from build123d import *

# Parameters (mm, degrees)
SKETCH1_W           = 50.8
SKETCH1_H           = 76.2
SKETCH1_W_2         = 44.45
SKETCH1_H_2         = 69.85
BOSS_EXTRUDE1_DEPTH = 965.2
CUT_EXTRUDE1_REACH  = 969.287
SKETCH4_R           = 14.224
SKETCH5_R           = 2.50063
CUT_EXTRUDE2_DEPTH  = 3.175


with BuildPart() as part:
    # Sketch1 → Boss-Extrude1 (new body)
    with BuildSketch(Plane.XY):
        Rectangle(SKETCH1_W, SKETCH1_H)
        Rectangle(SKETCH1_W_2, SKETCH1_H_2, mode=Mode.SUBTRACT)
    extrude(amount=BOSS_EXTRUDE1_DEPTH)

    # Cut-Extrude1: up to this face of the body (flat: up to its plane)
    cut_extrude1_end = Plane(part.part.faces().sort_by_distance((-25.4, 0, 482.6))[0])
    # Sketch4 → Cut-Extrude1 (cut, up to the picked face)
    with BuildSketch(Plane(origin=(25.4, 0, 0), x_dir=(0, 0, -1), z_dir=(1, 0, 0)), mode=Mode.PRIVATE) as cut_extrude1_sk1:
        with Locations(Location((-703.246600733, 0, 0), (0, 0, 90))):
            Circle(SKETCH4_R)
    cut_extrude1_tool1 = split(extrude(cut_extrude1_sk1.sketch, amount=-CUT_EXTRUDE1_REACH, mode=Mode.PRIVATE), bisect_by=cut_extrude1_end, keep=Keep.BOTH, mode=Mode.PRIVATE)
    # Sketch4 → Cut-Extrude1 (cut, up to the picked face)
    with BuildSketch(Plane(origin=(25.4, 0, 0), x_dir=(0, 0, -1), z_dir=(1, 0, 0)), mode=Mode.PRIVATE) as cut_extrude1_sk2:
        with Locations(Location((-190.549048411, 0, 0), (0, 0, 90))):
            Circle(SKETCH4_R)
    cut_extrude1_tool2 = split(extrude(cut_extrude1_sk2.sketch, amount=-CUT_EXTRUDE1_REACH, mode=Mode.PRIVATE), bisect_by=cut_extrude1_end, keep=Keep.BOTH, mode=Mode.PRIVATE)
    # Sketch4 → Cut-Extrude1 (cut, up to the picked face)
    with BuildSketch(Plane(origin=(25.4, 0, 0), x_dir=(0, 0, -1), z_dir=(1, 0, 0)), mode=Mode.PRIVATE) as cut_extrude1_sk3:
        with Locations(Location((-446.897824572, 0, 0), (0, 0, 90))):
            Circle(SKETCH4_R)
    cut_extrude1_tool3 = split(extrude(cut_extrude1_sk3.sketch, amount=-CUT_EXTRUDE1_REACH, mode=Mode.PRIVATE), bisect_by=cut_extrude1_end, keep=Keep.BOTH, mode=Mode.PRIVATE)
    add(cut_extrude1_tool1.solids().sort_by(Axis((25.4, 0, 703.246601), (-1, 0, 0)))[0], mode=Mode.SUBTRACT)
    add(cut_extrude1_tool2.solids().sort_by(Axis((25.4, 0, 190.549048), (-1, 0, 0)))[0], mode=Mode.SUBTRACT)
    add(cut_extrude1_tool3.solids().sort_by(Axis((25.4, 0, 446.897825), (-1, 0, 0)))[0], mode=Mode.SUBTRACT)

    # Sketch5 → Cut-Extrude2 (cut)
    with BuildSketch(Plane(origin=(0, 38.1, 0), x_dir=(1, 0, 0), z_dir=(0, 1, 0))):
        with Locations(Location((8.89, -571.614708402, 0), (0, 0, 270))):
            Circle(SKETCH5_R)
        with Locations(Location((19.05, -571.614708402, 0), (0, 0, 270))):
            Circle(SKETCH5_R)
        with Locations((19.05, -320.473808194)):
            Circle(SKETCH5_R)
        with Locations((8.89, -320.473808194)):
            Circle(SKETCH5_R)
    extrude(amount=-CUT_EXTRUDE2_DEPTH, mode=Mode.SUBTRACT)


solid = part.part
The listing builds one solid part. Answer for the finished solid, in the listing's coordinates (mm). A direction names the side the tool comes from. Coordinates: 2 decimals unless noted, no trailing zeros. Loops run counter-clockwise (first coordinate to the right, second up) from the corner with the lowest first, then second, coordinate; pieces in that order, holes last.
1) Find section B-B on x = -4.5. Write down the section's boundary in (y, z) (3 decimals), then the cut area to 3 significant figures.
2) Determine the mould class of faces 1 (the face through (0, 34.925, 476)), 2 (the face through (0, 38.1, 476)), 3 (the face through (-23, 3, 965.2)), 4 (the face through (23.83, -3.08, 433.01)) for opening direction Y: pulls with the +Y half, pulls with the -Y half, needs draft (parallel to the pull), parting line crosses it, or undercut.
3) Find section A-A on y = 23.5. Write down the section's boundary in (x, z) (3 decimals), then the cut area to 3 significant figures.
4) A tool of negligible diameter and unlimited length cuts with its end or side. For faces 5 (the face through (0, -34.925, 476)), 6 (the face through (23.835, -1.852, 204.652)), from which of +Z, -Z, +X, -X, +Y, -Y can it reach the whole face along a straight path? Write none if from no direction.
5) A flat-ended cylindrical pin translates along its axis: pin 1 Ø23 at (y, z) = (0, 446.9) entering from -X. Find the tip coordinate at first contact, or state that the pin passes through.
6) Find the intervals of material crossed by L1, parallel to Z at x = -24, y = 0; L2, parallel to X at y = 1.5, z = 95 (3 decimals); L3, parallel to Y at x = 14.5, z = 254 (3 decimals), in increasing order.
7) Find section C-C on z = 490.5. Write down the section's boundary in (x, y) (3 decimals), then the cut area to 3 significant figures.
Values:
1. outline: (-38.1, 0) - (-34.925, 0) - (-34.925, 965.2) - (-38.1, 965.2) - close; (34.925, 0) - (38.1, 0) - (38.1, 965.2) - (34.925, 965.2) - close
1. area: 6,130 mm2
2. face 1: undercut
2. face 2: pulls with the +Y half
2. face 3: needs draft
2. face 4: undercut
3. outline: (-25.4, 0) - (-22.225, 0) - (-22.225, 965.2) - (-25.4, 965.2) - close; (22.225, 0) - (25.4, 0) - (25.4, 965.2) - (22.225, 965.2) - close
3. area: 6,130 mm2
4. face 5: +Z, -Z
4. face 6: +X, -X
5. pin 1: passes through
6. L1: z = 0 to 176.33, 204.77 to 432.67, 461.12 to 689.02, 717.47 to 965.2
6. L2: x = -25.4 to -22.225, 22.225 to 25.4
6. L3: y = -38.1 to -34.925, 34.925 to 38.1
7. outline: (-25.4, -38.1) - (25.4, -38.1) - (25.4, 38.1) - (-25.4, 38.1) - close; hole (-22.225, -34.925) - (22.225, -34.925) - (22.225, 34.925) - (-22.225, 34.925) - close
7. area: 766 mm2
